Could you check a few things on this model? Use its own coordinates, in mm. A direction names the side the tool comes from. Give positions to 0.01 mm unless a question says otherwise; leave off trailing zeros. Order: outer loops, then holes, each group sorted by start corner. A loop starts at its lowest first (then second) coordinate and runs counter-clockwise, first axis right, second up. Notation, with made-up numbers: (7.25, -35) -> (34.25, -35) arc R21 cw to (34.25, -4) -> close; hole circle Ø1 at (34, 48.25). An arc over 180 degrees is marked (long way). Answer as CSV lines item,"result". Start each with the question number.
(1) On a 3-axis mill with a long thin cutter (end or side, diameter ignored), from which of +Z, -Z, +X, -X, +Y, -Y can I reach the whole of each face in a straight line? I mean faces 4 (the face through (-0.1, -22.5, 2174.6)), 5 (the face through (0, 22.225, 1085)). Say none if no direction works.
(2) I want a section at C-C (z = 1554). Please give me the cut outline in (x, y) (3 decimals).
(3) I want a section at A-A (y = -8). Please give me the cut outline in (x, z) (3 decimals), plus the area to 3 significant figures.
(4) We'd pull the mould along Y, two halves only. Please class faces 1 (the face through (-22.225, 0, 1085)), 2 (the face through (-0.1, -22.5, 25.4)), 3 (the face through (0, -25.4, 1085)): released by +Y, released by -Y, zero draft, split by the parting line, or undercut.
(5) I need wall thicknesses on L1, parallel to X at y = -6, z = 1933 (3 decimals); L2, parallel to X at y = 20, z = 394. Which ranges of each line are inside material? Lowest first, please.
Autodesk Inventor part; units mm, degrees
ref_plane "Plano inicial" through (0, 0, 25.4) normal (0, 0, 1) x (1, 0, 0)
ref_plane "Plano final" through (0, 0, 2174.6) normal (0, 0, 1) x (1, 0, 0)
ref_plane "Plano de trabajo4" through (-2980.95, 0, 2174.6) normal (0, 0, 1) x (1, 0, 0)
ref_plane "Plano inicial" through (0, 0, 25.4) normal (0, 0, 1) x (1, 0, 0)
ref_plane "Plano final" through (0, 0, 2174.6) normal (0, 0, 1) x (1, 0, 0)
sketch "Boceto" plane through (0, 0, 0) normal (0, 0, 1) x (1, 0, 0)
  line L0 (-25.4, -19.05) -> (-25.4, 19.05)
  line L1 (-19.05, 25.4) -> (19.05, 25.4)
  line L2 (25.4, 19.05) -> (25.4, -19.05)
  line L3 (19.05, -25.4) -> (-19.05, -25.4)
  arc A0 (-25.4, -19.05) -> (-19.05, -25.4) centre (-19.05, -19.05) ccw
  arc A1 (-19.05, 25.4) -> (-25.4, 19.05) centre (-19.05, 19.05) ccw
  arc A2 (25.4, 19.05) -> (19.05, 25.4) centre (19.05, 19.05) ccw
  arc A3 (19.05, -25.4) -> (25.4, -19.05) centre (19.05, -19.05) ccw
  arc A4 (-19.05, 22.225) -> (-22.225, 19.05) centre (-19.05, 19.05) ccw
  line L4 (-19.05, 22.225) -> (19.05, 22.225)
  arc A5 (22.225, 19.05) -> (19.05, 22.225) centre (19.05, 19.05) ccw
  line L5 (22.225, 19.05) -> (22.225, -19.05)
  arc A6 (19.05, -22.225) -> (22.225, -19.05) centre (19.05, -19.05) ccw
  line L6 (19.05, -22.225) -> (-19.05, -22.225)
  arc A7 (-22.225, -19.05) -> (-19.05, -22.225) centre (-19.05, -19.05) ccw
  line L7 (-22.225, -19.05) -> (-22.225, 19.05)
  line L8 (0, 37.4012) -> (0, -37.4012) construction
  line L9 (-37.4012, 0) -> (37.4012, 0) construction
  dimension "d10" = 50.8
  dimension "d11" = 50.8
  dimension "d12" = 3.175
  dimension "d15" = 25.4
  dimension "d16" = 25.4
  dimension "d17" = 6.35
extrude "Cuerpo" add sketch "Boceto" along normal up to surface (2149.2 mm away) from surface at 25.4
sketch "Sketch3" plane through (0, 0, 0) normal (0, 0, 1) x (1, 0, 0)
  line L0 (0, 0) -> (10, 0)
ref_plane "Work Plane3" through (0, 0, 0) normal (0, -1, 0) x (1, 0, 0)
ref_plane "Plano de trabajo4" through (-2980.95, 0, 2174.6) normal (0, 0, 1) x (1, 0, 0)
split "Dividir1" plane through (-2980.95, 0, 2174.6) removes the side toward (0, 0, 1)
ref_plane "Plano de trabajo5" through (-3000, -19.05, 25.4) normal (0, 0, -1) x (-1, 0, 0)
split "Dividir2" plane through (-3000, -19.05, 25.4) removes the side toward (0, 0, -1)
ref_plane "Plano de trabajo6" through (-2980.95, -2890, 25.4) normal (0, 0, -1) x (-1, 0, 0)
split "Dividir3" plane through (-2980.95, -2890, 25.4) removes the side toward (0, 0, -1)
sketch "Sketch4" plane through (0, 0, 0) normal (0, -1, 0) x (1, 0, 0)
  line L0 (-2, 25.4) -> (12, 25.4)
  line L1 (-2, 2174.6) -> (12, 2174.6)
  dimension "d19" = 2149.2
equation "\"d10\" = G_H"
equation "\"d11\" = G_W"
equation "\"d12\" = G_T"
equation "\"d15\" = 0.5 * d10"
equation "\"d16\" = 0.5 * d11"
equation "\"d17\" = G_IR"
equation "\"d3\" = G_L"
equation "\"G_W\" = 50.8"
equation "\"G_H\" = 50.8"
equation "\"G_T\" = 3.175"
equation "\"G_IR\" = 6.35"
equation "\"G_L\" = d19"
equation "\"G_OFFSET_START\" = -25.4"
equation "\"G_OFFSET_END\" = -25.4"
equation "\"d13\" = -G_OFFSET_START"
equation "\"d14\" = G_OFFSET_END + B_L"
equation "\"B_L\" = 2200"
properties part number "AISC - 2 x 2 x 1/8 - 84,614" material "Acero, suave"
Final values:
1,face 4,"+Z, +X, -X, +Y, -Y"
1,face 5,"+Z, -Z"
2,outline,"(-25.4, -19.05) arc R6.35 ccw to (-19.05, -25.4) -> (19.05, -25.4) arc R6.35 ccw to (25.4, -19.05) -> (25.4, 19.05) arc R6.35 ccw to (19.05, 25.4) -> (-19.05, 25.4) arc R6.35 ccw to (-25.4, 19.05) -> close; hole (-22.225, -19.05) arc R3.175 ccw to (-19.05, -22.225) -> (19.05, -22.225) arc R3.175 ccw to (22.225, -19.05) -> (22.225, 19.05) arc R3.175 ccw to (19.05, 22.225) -> (-19.05, 22.225) arc R3.175 ccw to (-22.225, 19.05) -> close"
3,outline,"(-25.4, 25.4) -> (-22.225, 25.4) -> (-22.225, 2174.6) -> (-25.4, 2174.6) -> close; (22.225, 25.4) -> (25.4, 25.4) -> (25.4, 2174.6) -> (22.225, 2174.6) -> close"
3,area,"13,600 mm²"
4,face 1,"undercut"
4,face 2,"zero draft"
4,face 3,"released by -Y"
5,L1,"-25.4 to -22.225, 22.225 to 25.4"
5,L2,"-25.33 to -22.08, 22.08 to 25.33"
